Here's how the part is built. I have some questions about the finished solid (model axes, mm). Give positions to 0.01 mm unless a question says otherwise; leave off trailing zeros. Write each loop counter-clockwise with the first axis right and the second up, starting at its lowest first coordinate (ties: lowest second). Pieces come first, ordered by that corner, then holes. Notation, with made-up numbers: (43.5, 45) -> (87.5, 45) arc R23 cw to (87.5, 65) -> close; hole circle Ø1 at (13.5, -23). An arc over 180 degrees is marked (long way). Return JSON: item names as keys, results as strings.
from build123d import *

# Parameters (mm, degrees)
SKETCH1_W           = 146.685
SKETCH1_H           = 212.725
SKETCH1_R           = 2.4892
BOSS_EXTRUDE1_DEPTH = 1.5875
FILLET1_R           = 3.175
SKETCH2_R           = 1.3
CUT_EXTRUDE1_DEPTH  = 130.236931012
SKETCH3_R           = 1.3
CUT_EXTRUDE2_DEPTH  = 130.236931012
SKETCH4_R           = 2.4892
CUT_EXTRUDE3_DEPTH  = 130.236931012
CUT_EXTRUDE4_REACH  = 131.237
SKETCH5_R           = 2.4892


with BuildPart() as part:
    # Sketch1 → Boss-Extrude1 (new, symmetric)
    with BuildSketch(Plane(origin=(0, 0, 0), x_dir=(1, 0, 0), z_dir=(0, 1, 0))):
        Rectangle(SKETCH1_W, SKETCH1_H)
        with Locations(Location((-60.6425, 93.6625, 0), (0, 0, 270))):
            Circle(SKETCH1_R, mode=Mode.SUBTRACT)
        with Locations(Location((60.6425, 93.6625, 0), (0, 0, 270))):
            Circle(SKETCH1_R, mode=Mode.SUBTRACT)
        with Locations(Location((60.6425, -93.6625, 0), (0, 0, 270))):
            Circle(SKETCH1_R, mode=Mode.SUBTRACT)
        with Locations(Location((-60.6425, -93.6625, 0), (0, 0, 270))):
            Circle(SKETCH1_R, mode=Mode.SUBTRACT)
    extrude(amount=BOSS_EXTRUDE1_DEPTH, both=True)

    # Fillet1
    fillet1_edges = [part.edges().sort_by_distance(p)[0] for p in [
        (73.3425, 0, 106.3625),
        (-73.3425, 0, 106.3625),
        (-73.3425, 0, -106.3625),
        (73.3425, 0, -106.3625),
    ]]
    fillet(fillet1_edges, radius=FILLET1_R)

    # Sketch2 → Cut-Extrude1 (cut, through all)
    with BuildSketch(Plane(origin=(0, 1.5875, 0), x_dir=(1, 0, 0), z_dir=(0, 1, 0))):
        with Locations(Location((40, 13.8625, 0), (0, 0, 270))):
            Circle(SKETCH2_R)
        with Locations(Location((40, 71.8625, 0), (0, 0, 270))):
            Circle(SKETCH2_R)
        with Locations(Location((-46, 71.8625, 0), (0, 0, 270))):
            Circle(SKETCH2_R)
        with Locations(Location((-46, 13.8625, 0), (0, 0, 270))):
            Circle(SKETCH2_R)
        with Locations(Location((46, 13.8625, 0), (0, 0, 270))):
            Circle(SKETCH2_R)
        with Locations(Location((46, 71.8625, 0), (0, 0, 270))):
            Circle(SKETCH2_R)
        with Locations(Location((-40, 71.8625, 0), (0, 0, 270))):
            Circle(SKETCH2_R)
        with Locations(Location((-40, 13.8625, 0), (0, 0, 270))):
            Circle(SKETCH2_R)
    extrude(amount=-CUT_EXTRUDE1_DEPTH, mode=Mode.SUBTRACT)

    # Sketch3 → Cut-Extrude2 (cut, through all)
    with BuildSketch(Plane(origin=(0, 1.5875, 0), x_dir=(1, 0, 0), z_dir=(0, 1, 0))):
        with Locations(Location((67.75, 70.962500061, 0), (0, 0, 270))):
            Circle(SKETCH3_R)
        with Locations(Location((-67.75, 70.962500061, 0), (0, 0, 270))):
            Circle(SKETCH3_R)
        with Locations(Location((-67.75, 27.462499939, 0), (0, 0, 270))):
            Circle(SKETCH3_R)
        with Locations(Location((67.75, 27.462499939, 0), (0, 0, 270))):
            Circle(SKETCH3_R)
    extrude(amount=-CUT_EXTRUDE2_DEPTH, mode=Mode.SUBTRACT)

    # Sketch4 → Cut-Extrude3 (cut, through all)
    with BuildSketch(Plane(origin=(0, 1.5875, 0), x_dir=(1, 0, 0), z_dir=(0, 1, 0))):
        with Locations(Location((-40.3225, -61.9125, 0), (0, 0, 270))):
            Circle(SKETCH4_R)
        with Locations(Location((40.3225, -61.9125, 0), (0, 0, 270))):
            Circle(SKETCH4_R)
    extrude(amount=-CUT_EXTRUDE3_DEPTH, mode=Mode.SUBTRACT)

    # Sketch5 → Cut-Extrude4 (cut, up to next)
    with BuildSketch(Plane(origin=(0, 1.5875, 0), x_dir=(1, 0, 0), z_dir=(0, 1, 0)), mode=Mode.PRIVATE) as cut_extrude4_sk1:
        with Locations(Location((17.4625, -38.1, 0), (0, 0, 270))):
            Circle(SKETCH5_R)
    cut_extrude4_tool1 = extrude(cut_extrude4_sk1.sketch, amount=-CUT_EXTRUDE4_REACH, mode=Mode.PRIVATE) & part.part
    # Sketch5 → Cut-Extrude4 (cut, up to next)
    with BuildSketch(Plane(origin=(0, 1.5875, 0), x_dir=(1, 0, 0), z_dir=(0, 1, 0)), mode=Mode.PRIVATE) as cut_extrude4_sk2:
        with Locations(Location((17.4625, -3.175, 0), (0, 0, 270))):
            Circle(SKETCH5_R)
    cut_extrude4_tool2 = extrude(cut_extrude4_sk2.sketch, amount=-CUT_EXTRUDE4_REACH, mode=Mode.PRIVATE) & part.part
    # Sketch5 → Cut-Extrude4 (cut, up to next)
    with BuildSketch(Plane(origin=(0, 1.5875, 0), x_dir=(1, 0, 0), z_dir=(0, 1, 0)), mode=Mode.PRIVATE) as cut_extrude4_sk3:
        with Locations(Location((-17.4625, -3.175, 0), (0, 0, 270))):
            Circle(SKETCH5_R)
    cut_extrude4_tool3 = extrude(cut_extrude4_sk3.sketch, amount=-CUT_EXTRUDE4_REACH, mode=Mode.PRIVATE) & part.part
    # Sketch5 → Cut-Extrude4 (cut, up to next)
    with BuildSketch(Plane(origin=(0, 1.5875, 0), x_dir=(1, 0, 0), z_dir=(0, 1, 0)), mode=Mode.PRIVATE) as cut_extrude4_sk4:
        with Locations(Location((-17.4625, -38.1, 0), (0, 0, 270))):
            Circle(SKETCH5_R)
    cut_extrude4_tool4 = extrude(cut_extrude4_sk4.sketch, amount=-CUT_EXTRUDE4_REACH, mode=Mode.PRIVATE) & part.part
    add(cut_extrude4_tool1.solids().sort_by_distance((17.4625, 1.5875, 38.1))[0], mode=Mode.SUBTRACT)
    add(cut_extrude4_tool2.solids().sort_by_distance((17.4625, 1.5875, 3.175))[0], mode=Mode.SUBTRACT)
    add(cut_extrude4_tool3.solids().sort_by_distance((-17.4625, 1.5875, 3.175))[0], mode=Mode.SUBTRACT)
    add(cut_extrude4_tool4.solids().sort_by_distance((-17.4625, 1.5875, 38.1))[0], mode=Mode.SUBTRACT)


solid = part.part
1. Suppose I cut it at A-A, the plane z = 38.1. List the corners of the cut face in (x, y) for me, and give its area (3 significant figures).
Taken from the geometry:
{"outline": "(-73.34, -1.59) -> (-19.95, -1.59) -> (-19.95, 1.59) -> (-73.34, 1.59) -> close; (-14.97, -1.59) -> (14.97, -1.59) -> (14.97, 1.59) -> (-14.97, 1.59) -> close; (19.95, -1.59) -> (73.34, -1.59) -> (73.34, 1.59) -> (19.95, 1.59) -> close", "area": "434 mm²"}
2. For pin 1 Ø2 at (x, z) = (-67.75, -27.46) entering from +Y, with a flat end and sliding along its axis, tell me the tip position at first contact or that it passes through.
Taken from the geometry:
{"pin 1": "passes through"}
3. If we mould it in two halves opening along X, with no side actions, what happens to faces 1 (the face through (17.572, 0.022, 35.613)), 2 (the face through (-1, -1.588, -1))? For each: released by +X, released by -X, zero draft, split by the parting line, or undercut.
Taken from the geometry:
{"face 1": "undercut", "face 2": "zero draft"}
4. If I drill on line 1 (Z direction, x = 67.75, y = 0); line 2 (X direction, y = -0.15, z = -13.5); line 3 (X direction, y = 1.35, z = 2), over which ranges is the centre line in solid material (lowest first)? Write a range as [from, to].
Taken from the geometry:
{"line 1": "z = [-106.36, -72.26], [-69.66, -28.76], [-26.16, 106.36]", "line 2": "x = [-73.34, -47.25], [-44.75, -41.25], [-38.75, 38.75], [41.25, 44.75], [47.25, 73.34]", "line 3": "x = [-73.34, -19.66], [-15.27, 15.27], [19.66, 73.34]"}
